from build123d import *

# Parameters (mm, degrees)
F1_W     = 50
F1_H     = 50
F1_R     = 11.7
F1_R_2   = 10.1
F2_DEPTH = 1.6
F5_DEPTH = 20
F3_R     = 2
F4_SIZE  = 0.3


with BuildPart() as f2:
    # F1 (on Top) → F2 (new body)
    with BuildSketch(Plane.XY):
        Rectangle(F1_W, F1_H)
        Circle(F1_R, mode=Mode.SUBTRACT)
        Circle(F1_R)
        Circle(F1_R_2, mode=Mode.SUBTRACT)
        Circle(F1_R_2)
    extrude(amount=F2_DEPTH)

    # F1 (on Top) → F5 (join)
    with BuildSketch(Plane.XY):
        Circle(F1_R)
        Circle(F1_R_2, mode=Mode.SUBTRACT)
    extrude(amount=F5_DEPTH)

    # F3
    f3_edges = [f2.edges().sort_by_distance(p)[0] for p in [
        (25, 25, 0.8),
        (25, -25, 0.8),
        (-25, -25, 0.8),
        (-25, 25, 0.8),
    ]]
    fillet(f3_edges, radius=F3_R)

    # F4
    f4_edges = [f2.edges().sort_by_distance(p)[0] for p in [
        (0, 25, 1.6),
        (24.414214, 24.414214, 1.6),
        (-24.414214, 24.414214, 1.6),
        (25, 0, 1.6),
        (-25, 0, 1.6),
        (24.414214, -24.414214, 1.6),
        (-24.414214, -24.414214, 1.6),
        (0, -25, 1.6),
        (-11.7, 0, 1.6),
        (0, 25, 0),
        (24.414214, 24.414214, 0),
        (-24.414214, 24.414214, 0),
        (25, 0, 0),
        (-25, 0, 0),
        (24.414214, -24.414214, 0),
        (-24.414214, -24.414214, 0),
        (0, -25, 0),
        (-10.1, 0, 20),
        (-11.7, 0, 20),
        (-10.1, 0, 1.6),
    ]]
    chamfer(f4_edges, length=F4_SIZE)


solid = f2.part
Part model, mm, in its own coordinate system. A direction names the side the tool comes from. Coordinates: 2 decimals unless noted, no trailing zeros. Loops run counter-clockwise (first coordinate to the right, second up) from the corner with the lowest first, then second, coordinate; pieces in that order, holes last. Notation, with made-up numbers: M -3.5,15.25 L 8.5,15.25 A20 ccw 8.5,34.25 Z; hole C -13,33.5 d4. An arc over 180 degrees is marked long. Use a Markdown table: item, result. Add a question column.
Q1. Cut at C-C (z = 2.5). Write the cut outline in (x, y), and give its area (3 significant figures).
Q2. Probe L1, parallel to Y at x = 0, z = 13.5; L2, parallel to Z at x = -12, y = 1.5. List the from-to ranges inside material, lowest first.
Q3. Pin check, flat tips, straight feed: P1, Ø10, axis at y = 15, z = 14, coming from the +X side; P2, Ø6, axis at x = 3.5, y = 1.5, coming from the +Z side; P3, Ø12, axis at x = 11, z = 14, coming from the +Y side. Stop position of each tip, or through.
Q4. Cut at A-A (y = 0). Write the cut outline in (x, z), and give its area (3 significant figures).
Q5. Mould opens along Y. For faces 3 (the flat face through (0, 0, 1.6)), 4 (the conical face through (24.27, 24.3, 0.12)), 5 (the cylindrical face through (-24.43, -24.4, 0.81)) say: +Y half, -Y half, draft (parallel to the pull), parting line (faces both ways), or undercut.
Q6. Cut at B-B (x = 17.5). Write the cut outline in (y, z), and give its area (3 significant figures).
Q7. Which spindle directions (+Z, -Z, +X, -X, +Y, -Y) get a long thin tool onto all of the face, cutting with end or side? Do faces 1 (the cylindrical face through (9.634, 3.034, 10.675)), 2 (the flat face through (0, 0, 0)). Say none if no direction does.
Worked out:
| question | item | result |
|---|---|---|
| 1 | outline | C 0,0 d23.4; hole C 0,0 d20.2 |
| 1 | area | 110 mm2 |
| 2 | L1 | y = -11.7 to -10.1, 10.1 to 11.7 |
| 2 | L2 | z = 0 to 1.6 |
| 3 | P1 | stops at x = 6.07 |
| 3 | P2 | stops at z = 1.6 |
| 3 | P3 | stops at y = 10.58 |
| 4 | outline | M -25,0.3 L -24.7,0 L 24.7,0 L 25,0.3 L 25,1.3 L 24.7,1.6 L 12,1.6 L 11.7,1.9 L 11.7,19.7 L 11.4,20 L 10.4,20 L 10.1,19.7 L 10.1,1.9 L 9.8,1.6 L -9.8,1.6 L -10.1,1.9 L -10.1,19.7 L -10.4,20 L -11.4,20 L -11.7,19.7 L -11.7,1.9 L -12,1.6 L -24.7,1.6 L -25,1.3 Z |
| 4 | area | 139 mm2 |
| 5 | face 3 | undercut |
| 5 | face 4 | +Y half |
| 5 | face 5 | -Y half |
| 6 | outline | M -25,0.3 L -24.7,0 L 24.7,0 L 25,0.3 L 25,1.3 L 24.7,1.6 L -24.7,1.6 L -25,1.3 Z |
| 6 | area | 79.8 mm2 |
| 7 | face 1 | +Z |
| 7 | face 2 | -Z, +X, -X, +Y, -Y |
